Build history of the part. All positions in model axes, mm. A direction names the side the tool comes from. Give positions to 0.01 mm unless a question says otherwise; leave off trailing zeros. Order: outer loops, then holes, each group sorted by start corner. A loop starts at its lowest first (then second) coordinate and runs counter-clockwise, first axis right, second up. Notation, with made-up numbers: M -3,67 L 48,67 A21 ccw 48,71 Z; hole C 85,67 d7. An arc over 180 degrees is marked long. Use CSV: the item, a comma, the result in double quotes. Start each with the question number.
Item 1: Band-saw the part on D-D on x = -1. Write the cut outline in (y, z).
Item 2: Wall check: line 1 along Z through (x, y) = (1.5, -0.25); line 2 along X through (y, z) = (-4, 2.25); line 3 along Z through (x, y) = (6.5, 0). Give the ranges that are in metal, low to high.
Item 3: Band-saw the part on B-B on y = 0. Write the cut outline in (x, z), plus the area to 3 significant figures.
Item 4: Band-saw the part on C-C on x = 5.5. Write the cut outline in (y, z), plus the area to 3 significant figures.
Item 5: Which spindle directions (+Z, -Z, +X, -X, +Y, -Y) get a long thin tool onto all of the face, cutting with end or side? Do faces 4 (the flat face through (7, 0, 3.8)), 5 (the flat face through (-4.5, 0, 0)), 6 (the flat face through (7, 0, -3.8)), 7 (the cylindrical face through (8.2, -0.07, -2.79)), 8 (the flat face through (3, 3, 0)). Say none if no direction does.
Item 6: Pin check, flat tips, straight feed: P1, Ø6, axis at x = -1, z = 6, coming from the -Y side; P2, Ø2, axis at y = -5, z = -6, coming from the -X side; P3, Ø2, axis at y = -3.5, z = -5, coming from the +X side; P4, Ø5, axis at x = 8, y = 0.5, coming from the -Z side. Stop position of each tip, or through.
Item 7: Two-plate mould, pull along X, no slides. Class faces 1 (the flat face through (3, -3, 0)), 2 (the cylindrical face through (8.2, -0.07, 2.79)), 3 (the cylindrical face through (9.7, -0.1, 0)): pulls with the +X half, pulls with the -X half, needs draft (parallel to the pull), parting line crosses it, or undercut.
Item 8: Band-saw the part on A-A on z = 0. Write the cut outline in (x, y), plus the area to 3 significant figures.
from build123d import *

# Parameters (mm, degrees)
EXTRUDE_1_DEPTH = 1.8
SKETCH_4_W      = 1.5
SKETCH_4_H      = 2


with BuildPart() as part:
    # 草图1 → 旋转1 (revolve)
    with BuildSketch(Plane.XY, mode=Mode.PRIVATE) as revolve_1_sk:
        Polygon((-4.5, 7), (-4.5, 0), (0, 0), (0, 8), (-3.5, 8), align=None)
    revolve(revolve_1_sk.sketch.rotate(Axis((-4.5, 0, 0), (1, 0, 0)), 90), axis=Axis((-4.5, 0, 0), (1, 0, 0)))

    # 草图3 → 凸台-拉伸1 (add, symmetric)
    with BuildSketch(Plane.XY):
        with BuildLine():
            Line((0, -3), (6.7, -3))
            ThreePointArc((6.7, -3), (9.7, 0), (6.7, 3))
            Line((6.7, 3), (0, 3))
            Line((0, 3), (0, -3))
        make_face()
    extrude(amount=EXTRUDE_1_DEPTH, both=True)

    # 草图4 → 旋转2 (revolve)
    with BuildSketch(Plane(origin=(0, 0, 0), x_dir=(1, 0, 0), z_dir=(0, 1, 0)), mode=Mode.PRIVATE) as revolve_2_sk:
        with Locations((7.45, -2.8)):
            Rectangle(SKETCH_4_W, SKETCH_4_H)
    revolve_2 = revolve(revolve_2_sk.sketch.rotate(Axis((6.7, 0, 1.8), (0, 0, 1)), 180), axis=Axis((6.7, 0, 1.8), (0, 0, 1)))

    # 镜向1: 旋转2 across plane
    add(revolve_2.mirror(Plane.XY))


solid = part.part
Model answer:
1,outline,"C 0,0 d16"
2,line 1,"z = -1.8 to 1.8"
2,line 2,"x = -4.5 to 0"
2,line 3,"z = -3.8 to 3.8"
3,outline,"M -4.5,-7 L -3.5,-8 L 0,-8 L 0,-1.8 L 5.2,-1.8 L 5.2,-3.8 L 8.2,-3.8 L 8.2,-1.8 L 9.7,-1.8 L 9.7,1.8 L 8.2,1.8 L 8.2,3.8 L 5.2,3.8 L 5.2,1.8 L 0,1.8 L 0,8 L -3.5,8 L -4.5,7 Z"
3,area,"118 mm^2"
4,outline,"M -3,-1.8 L -0.9,-1.8 L -0.9,-3.8 L 0.9,-3.8 L 0.9,-1.8 L 3,-1.8 L 3,1.8 L 0.9,1.8 L 0.9,3.8 L -0.9,3.8 L -0.9,1.8 L -3,1.8 Z"
4,area,"28.8 mm^2"
5,face 4,"+Z, +X, +Y, -Y"
5,face 5,"+Z, -Z, -X, +Y, -Y"
5,face 6,"-Z, +X, +Y, -Y"
5,face 7,"-Z"
5,face 8,"+Z, -Z, +X, +Y"
6,P1,"stops at y = -7.42"
6,P2,"stops at x = -4.5"
6,P3,"stops at x = 0"
6,P4,"stops at z = -3.8"
7,face 1,"needs draft"
7,face 2,"undercut"
7,face 3,"pulls with the +X half"
8,outline,"M -4.5,-7 L -3.5,-8 L 0,-8 L 0,-3 L 6.7,-3 A3 ccw 6.7,3 L 0,3 L 0,8 L -3.5,8 L -4.5,7 Z"
8,area,"125 mm^2"
